Geometry: see drawing. Coordinates: mm, zero at the bounding-box minimum. Give positions to 0.01 mm unless a question says otherwise; leave off trailing zeros. Order: outer loops, then holes, each group sorted by start corner. A loop starts at its lowest first (then second) coordinate and runs counter-clockwise, first axis right, second up. Notation, with made-up numbers: M 57.5,48 L 64.5,48 A15 cw 64.5,76 Z; hole C 6,74 d5. An arc over 180 degrees is marked long. Use a Markdown table: item, result.
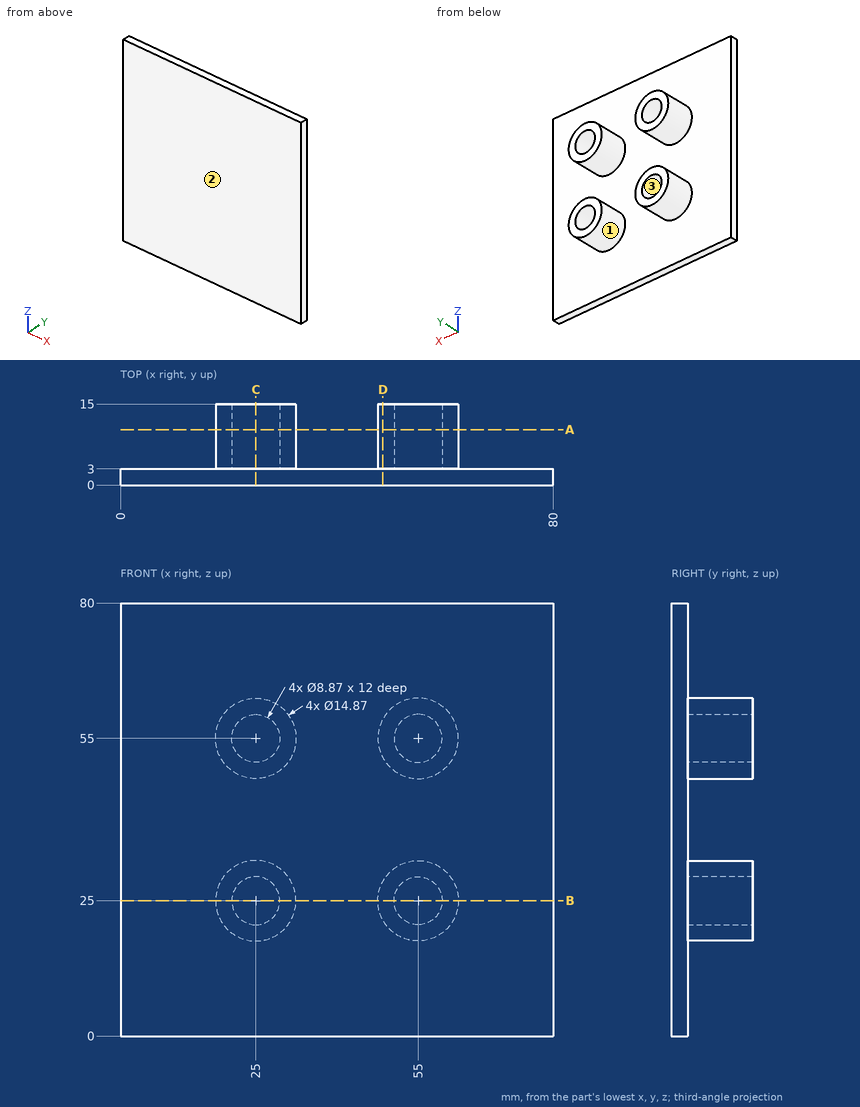
1) Cut plane A-A on y = 10.25. Return loops of the section in (x, z) (3 decimals).
Response values:
| item | result |
|---|---|
| outline | C 25,25 d14.87; C 25,55 d14.87; C 55,25 d14.87; C 55,55 d14.87; hole C 25,25 d8.87; hole C 25,55 d8.87; hole C 55,25 d8.87; hole C 55,55 d8.87 |
2) Cut plane C-C on x = 25. Return loops of the section in (y, z) (3 decimals).
Response values:
| item | result |
|---|---|
| outline | M 0,0 L 3,0 L 3,17.565 L 15,17.565 L 15,20.565 L 3,20.565 L 3,29.435 L 15,29.435 L 15,32.435 L 3,32.435 L 3,47.565 L 15,47.565 L 15,50.565 L 3,50.565 L 3,59.435 L 15,59.435 L 15,62.435 L 3,62.435 L 3,80 L 0,80 Z |
3) Material intervals for line 1 (X direction, y = 9.5, z = 55) (3 decimals); line 2 (Z direction, x = 54.5, y = 14.75); line 3 (X direction, y = 4.25, z = 57), sorted ascending. Write a range as from..to.
Response values:
| item | result |
|---|---|
| line 1 | x = 17.565..20.565, 29.435..32.435, 47.565..50.565, 59.435..62.435 |
| line 2 | z = 17.58..20.59, 29.41..32.42, 47.58..50.59, 59.41..62.42 |
| line 3 | x = 17.84..21.04, 28.96..32.16, 47.84..51.04, 58.96..62.16 |
4) Mould query, pull axis X, two halves, no side actions, for the marked faces 1, 2 and 3. Classes: released by +X, released by -X, zero draft, split by the parting line, or undercut.
Response values:
| item | result |
|---|---|
| face 1 | undercut |
| face 2 | zero draft |
| face 3 | undercut |
5) Cut plane D-D on x = 48.5. Return loops of the section in (y, z), and give its area (3 significant figures).
Response values:
| item | result |
|---|---|
| outline | M 0,0 L 3,0 L 3,21.39 L 15,21.39 L 15,28.61 L 3,28.61 L 3,51.39 L 15,51.39 L 15,58.61 L 3,58.61 L 3,80 L 0,80 Z |
| area | 413 mm² |
6) Cut plane B-B on z = 25. Return loops of the section in (x, y) (3 decimals).
Response values:
| item | result |
|---|---|
| outline | M 0,0 L 80,0 L 80,3 L 62.435,3 L 62.435,15 L 59.435,15 L 59.435,3 L 50.565,3 L 50.565,15 L 47.565,15 L 47.565,3 L 32.435,3 L 32.435,15 L 29.435,15 L 29.435,3 L 20.565,3 L 20.565,15 L 17.565,15 L 17.565,3 L 0,3 Z |
7) First-contact query: pin 1 Ø4.5 at (x, z) = (54.5, 53) entering from +Y; pin 2 Ø1 at (y, z) = (4, 16) entering from +X. Flat tips, straight axial feed; report the tip coordinate or a pass-through.
Response values:
| item | result |
|---|---|
| pin 1 | stops at y = 3 |
| pin 2 | passes through |
